from build123d import *

# Parameters (mm, degrees)
SKETCH1_W           = 68
SKETCH1_H           = 68
SKETCH1_W_2         = 2
SKETCH1_H_2         = 5
SKETCH1_R           = 5
BOSS_EXTRUDE1_DEPTH = 2
FILLET2_R           = 5
FILLET3_R           = 5
FILLET4_R           = 5
FILLET5_R           = 5


with BuildPart() as part:
    # Sketch1 → Boss-Extrude1 (new body)
    with BuildSketch(Plane.XY):
        Rectangle(SKETCH1_W, SKETCH1_H)
        with Locations((-29, -27.5)):
            Rectangle(SKETCH1_W_2, SKETCH1_H_2, mode=Mode.SUBTRACT)
        with Locations((0, -25)):
            Circle(SKETCH1_R, mode=Mode.SUBTRACT)
        with Locations((29, -27.5)):
            Rectangle(SKETCH1_W_2, SKETCH1_H_2, mode=Mode.SUBTRACT)
        with Locations((-28, 0)):
            Circle(SKETCH1_R, mode=Mode.SUBTRACT)
        with Locations((-29, 27.5)):
            Rectangle(SKETCH1_W_2, SKETCH1_H_2, mode=Mode.SUBTRACT)
        with BuildLine():
            ThreePointArc((-12, -2.5), (-14.5, 0), (-12, 2.5))
            Line((-12, 2.5), (-2.5, 2.5))
            Line((-2.5, 2.5), (-2.5, 12))
            ThreePointArc((-2.5, 12), (0, 14.5), (2.5, 12))
            Line((2.5, 12), (2.5, 2.5))
            Line((2.5, 2.5), (12, 2.5))
            ThreePointArc((12, 2.5), (14.5, 0), (12, -2.5))
            Line((12, -2.5), (2.5, -2.5))
            Line((2.5, -2.5), (2.5, -12))
            ThreePointArc((2.5, -12), (0, -14.5), (-2.5, -12))
            Line((-2.5, -12), (-2.5, -2.5))
            Line((-2.5, -2.5), (-12, -2.5))
        make_face(mode=Mode.SUBTRACT)
        with Locations((28, 0)):
            Circle(SKETCH1_R, mode=Mode.SUBTRACT)
        with Locations((0, 25)):
            Circle(SKETCH1_R, mode=Mode.SUBTRACT)
        with Locations((29, 27.5)):
            Rectangle(SKETCH1_W_2, SKETCH1_H_2, mode=Mode.SUBTRACT)
    extrude(amount=BOSS_EXTRUDE1_DEPTH)

    # Fillet2
    fillet2_edges = [part.edges().sort_by_distance(p)[0] for p in [
        (34, 34, 1),
    ]]
    fillet(fillet2_edges, radius=FILLET2_R)

    # Fillet3
    fillet3_edges = [part.edges().sort_by_distance(p)[0] for p in [
        (-34, 34, 1),
    ]]
    fillet(fillet3_edges, radius=FILLET3_R)

    # Fillet4
    fillet4_edges = [part.edges().sort_by_distance(p)[0] for p in [
        (-34, -34, 1),
    ]]
    fillet(fillet4_edges, radius=FILLET4_R)

    # Fillet5
    fillet5_edges = [part.edges().sort_by_distance(p)[0] for p in [
        (34, -34, 1),
    ]]
    fillet(fillet5_edges, radius=FILLET5_R)


solid = part.part
Input: part model. Units: mm. Frame: model coordinates. A direction names the side the tool comes from. Round coordinates to 2 decimals unless told otherwise and drop trailing zeros. Order: outer loops, then holes, each group sorted by start corner. A loop starts at its lowest first (then second) coordinate and runs counter-clockwise, first axis right, second up. Notation, with made-up numbers: (49, 85) - (108, 85) arc R13 cw to (108, 100) - close; hole circle Ø1 at (87, 9). An arc over 180 degrees is marked (long way). Use a Markdown table: item, result.
1. Material intervals for probe 1 along Y at (x, z) = (0, 1.2); probe 2 along Y at (x, z) = (-9.5, 0.4); probe 3 along X at (y, z) = (-1, 1.6), sorted ascending.
Evaluation:
| item | result |
|---|---|
| probe 1 | -34 to -30, -20 to -14.5, 14.5 to 20, 30 to 34 |
| probe 2 | -34 to -2.5, 2.5 to 34 |
| probe 3 | -34 to -32.9, -23.1 to -14.29, 14.29 to 23.1, 32.9 to 34 |
2. Section C-C on z = 0.95. State how many separate pieces and enclosed holes the cut face has, then the cut area to 3 significant figures.
Evaluation:
| item | result |
|---|---|
| separate pieces | 1 |
| enclosed holes | 9 |
| area | 3,990 mm^2 |
3. Access query for faces 1 (the face through (-7, 2.5, 1)), 2 (the face through (-33, -32, 1)). Directions: +Z, -Z, +X, -X, +Y, -Y. A direction counts if a zero-diameter tool reaches every point of the face in a straight line with its end or side. Return the directions, or none.
Evaluation:
| item | result |
|---|---|
| face 1 | +Z, -Z |
| face 2 | +Z, -Z, -X, -Y |
4. Section A-A on x = 9.5. Return the cut outline in (y, z).
Evaluation:
| item | result |
|---|---|
| outline | (-34, 0) - (-2.5, 0) - (-2.5, 2) - (-34, 2) - close; (2.5, 0) - (34, 0) - (34, 2) - (2.5, 2) - close |
5. Mould query, pull axis Y, two halves, no side actions, for faces 3 (the face through (0, 34, 1)), 4 (the face through (2.5, -7, 1)), 5 (the face through (0, -34, 1)). Classes: +Y half, -Y half, draft (parallel to the pull), parting line (faces both ways), or undercut.
Evaluation:
| item | result |
|---|---|
| face 3 | +Y half |
| face 4 | undercut |
| face 5 | -Y half |
6. Section D-D on x = -13.5. Return the cut outline in (y, z), then the cut area to 3 significant figures.
Evaluation:
| item | result |
|---|---|
| outline | (-34, 0) - (-2, 0) - (-2, 2) - (-34, 2) - close; (2, 0) - (34, 0) - (34, 2) - (2, 2) - close |
| area | 128 mm^2 |
7. Section B-B on x = 0. Return the cut outline in (y, z).
Evaluation:
| item | result |
|---|---|
| outline | (-34, 0) - (-30, 0) - (-30, 2) - (-34, 2) - close; (-20, 0) - (-14.5, 0) - (-14.5, 2) - (-20, 2) - close; (14.5, 0) - (20, 0) - (20, 2) - (14.5, 2) - close; (30, 0) - (34, 0) - (34, 2) - (30, 2) - close |
